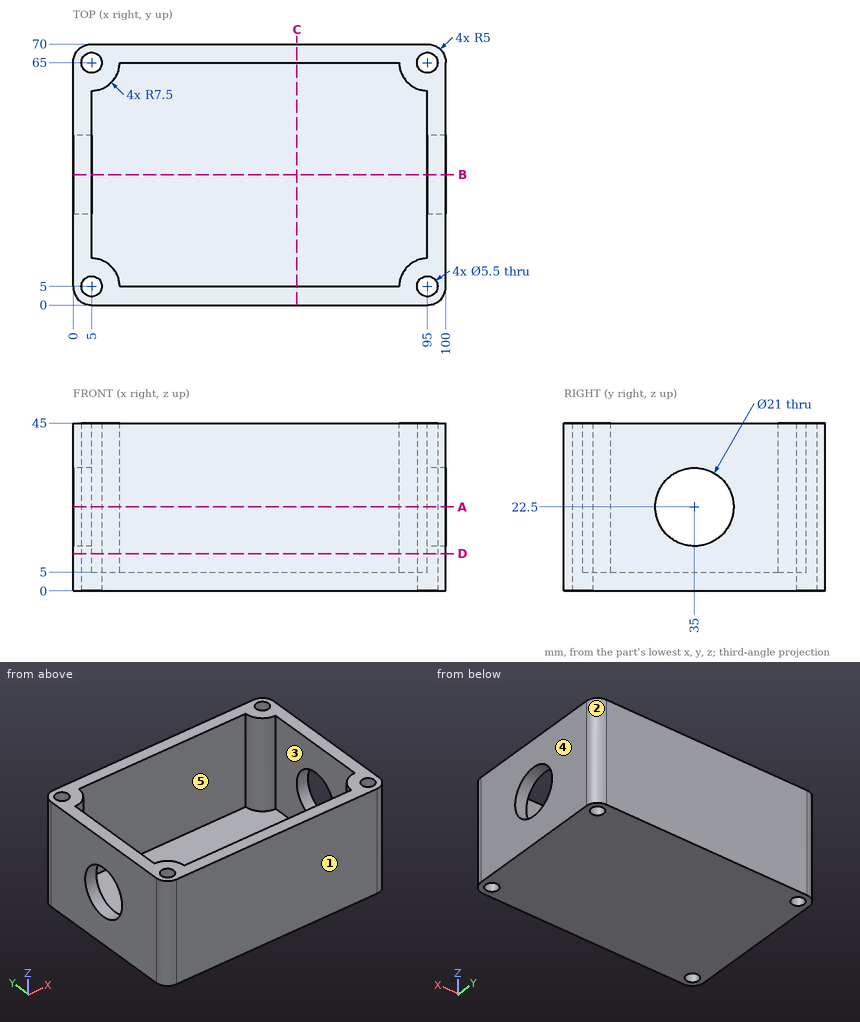
The figure shows three views and two pictorial views of one solid part (mm, origin at its lowest corner). Answer the questions. A direction names the side the tool comes from. Coordinates: 2 decimals unless noted, no trailing zeros. Loops run counter-clockwise (first coordinate to the right, second up) from the corner with the lowest first, then second, coordinate; pieces in that order, holes last. Notation, with made-up numbers: M -26,-3.75 L -9,-3.75 A20 ccw -9,26.25 Z; hole C -7.75,11.5 d5. An arc over 180 degrees is marked long. Use CSV: the item, a comma, the result in double quotes. Start each with the question number.
(1) For a pull along X with two mould halves and no side action, classify the marked faces 1, 2 and 3 as +X half, -X half, draft (parallel to the pull), parting line (faces both ways), or undercut.
(2) Find section C-C, the plane x = 60. Give the vertices of the cut face in (y, z), then the cut area to 3 significant figures.
(3) Find section D-D, the plane z = 10. Give the vertices of the cut face in (x, y), then the cut area to 3 significant figures.
(4) Given pin 1 Ø19 at (y, z) = (35, 22.5) entering from +X, flat-ended and moving along its own axis, determine where the tip first touches the part or whether it passes through.
(5) Consider line 1 (X direction, y = 23.5, z = 30.5); line 2 (Y direction, x = 80, z = 43); line 3 (Y direction, x = 96.5, z = 35.5). Determine where each line is inside the solid, lowest interval first.
(6) Find section B-B, the plane y = 35. Give the vertices of the cut face in (x, z).
(7) For the marked faces 4 and 5, determine the directions among +Z, -Z, +X, -X, +Y, -Y from which every point of the face is accessible in a straight line to the end or side of a thin tool.
(8) Find section A-A, the plane z = 22.5. Give the vertices of the cut face in (x, y), then the cut area to 3 significant figures.
Recorded:
1,face 1,"draft"
1,face 2,"+X half"
1,face 3,"undercut"
2,outline,"M 0,0 L 70,0 L 70,45 L 65,45 L 65,5 L 5,5 L 5,45 L 0,45 Z"
2,area,"750 mm^2"
3,outline,"M 0,5 A5 ccw 5,0 L 95,0 A5 ccw 100,5 L 100,65 A5 ccw 95,70 L 5,70 A5 ccw 0,65 Z; hole C 5,5 d5.5; hole C 5,65 d5.5; hole M 5,12.5 A7.5 cw 12.5,5 L 87.5,5 A7.5 cw 95,12.5 L 95,57.5 A7.5 cw 87.5,65 L 12.5,65 A7.5 cw 5,57.5 Z; hole C 95,5 d5.5; hole C 95,65 d5.5"
3,area,"1,660 mm^2"
4,pin 1,"passes through"
5,line 1,"x = 0 to 5, 95 to 100"
5,line 2,"y = 0 to 5, 65 to 70"
5,line 3,"y = 0.23 to 2.7, 7.3 to 62.7, 67.3 to 69.77"
6,outline,"M 0,0 L 100,0 L 100,12 L 95,12 L 95,5 L 5,5 L 5,12 L 0,12 Z; M 0,33 L 5,33 L 5,45 L 0,45 Z; M 95,33 L 100,33 L 100,45 L 95,45 Z"
7,face 4,"+Z, -Z, +X, +Y, -Y"
7,face 5,"+Z"
8,outline,"M 0,5 A5 ccw 5,0 L 95,0 A5 ccw 100,5 L 100,24.5 L 95,24.5 L 95,12.5 A7.5 ccw 87.5,5 L 12.5,5 A7.5 ccw 5,12.5 L 5,24.5 L 0,24.5 Z; M 0,45.5 L 5,45.5 L 5,57.5 A7.5 ccw 12.5,65 L 87.5,65 A7.5 ccw 95,57.5 L 95,45.5 L 100,45.5 L 100,65 A5 ccw 95,70 L 5,70 A5 ccw 0,65 Z; hole C 5,5 d5.5; hole C 5,65 d5.5; hole C 95,5 d5.5; hole C 95,65 d5.5"
8,area,"1,450 mm^2"
